from build123d import *

# Parameters (mm, degrees)
ESBO_O1_W                                = 150
ESBO_O1_H                                = 40
RESSALTO_EXTRUS_O1_DEPTH                 = 4
FILETE2_R                                = 15
BROCA_DE_ROSQUEAR_PARA_TARRAXA_DE_M201_D = 17.5


with BuildPart() as part:
    # Esboço1 → Ressalto-extrusão1 (new, symmetric)
    with BuildSketch(Plane.XY):
        with Locations((75, 20)):
            Rectangle(ESBO_O1_W, ESBO_O1_H)
    extrude(amount=RESSALTO_EXTRUS_O1_DEPTH, both=True)

    # Filete2
    filete2_edges = [part.edges().sort_by_distance(p)[0] for p in [
        (0, 0, 0),
        (0, 40, 0),
        (150, 40, 0),
        (150, 0, 0),
    ]]
    fillet(filete2_edges, radius=FILETE2_R)

    # Broca de rosquear para tarraxa de M201 (through all)
    with Locations(Plane.XY.offset(4)):
        with Locations((25, 20), (125, 20)):
            Hole(BROCA_DE_ROSQUEAR_PARA_TARRAXA_DE_M201_D / 2)


solid = part.part
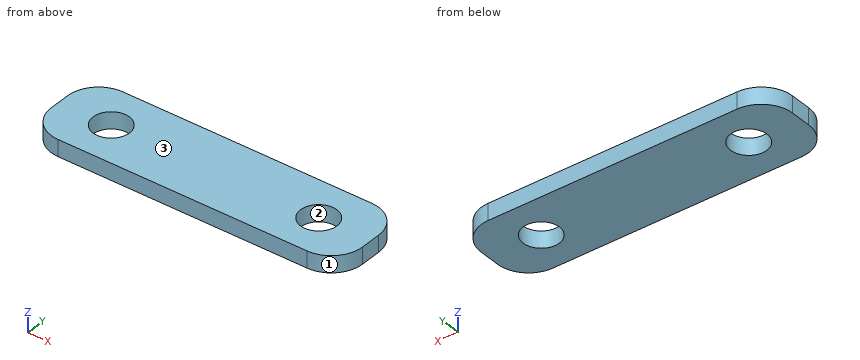
Could you check a few things on this model? Use its own coordinates, in mm. Face numbers are marked on the shaded views. Coordinates: 2 decimals unless noted, no trailing zeros. Order: outer loops, then holes, each group sorted by start corner. A loop starts at its lowest first (then second) coordinate and runs counter-clockwise, first axis right, second up. Notation, with made-up numbers: (-7, 23) - (47, 23) arc R22 ccw to (47, 56) - close; hole circle Ø11 at (50, -10). An arc over 180 degrees is marked (long way). Answer in a Markdown table with one row per item. Add a question column.
(1) I need wall thicknesses on L1, parallel to Y at x = 25, z = 1.5; L2, parallel to X at y = 25.5, z = -2.25; L3, parallel to X at y = 28, z = 0. Which ranges of each line are inside material? Lowest first, please.
(2) If we mould it in two halves opening along Y, with no side actions, what happens to the marked faces 1, 2 and 3? For each: released by +Y, released by -Y, zero draft, split by the parting line, or undercut.
(3) If we section it at A-A, the plane x = 125: Please give me the cut outline in (y, z), then the cut area to 3 significant figures.
(4) Will this pin go through, and if not, where does the flat tip stop? pin 1 (1 mm diameter, centred on y = 29.5, z = 1, fed in from -X).
(5) If we section it at B-B, the plane z = -0.5: Please give me the cut outline in (x, y), then the cut area to 3 significant figures.
(6) If we section it at C-C, the plane y = 20: Please give me the cut outline in (x, z).
(7) If we section it at D-D, the plane y = 3.5: Please give me the cut outline in (x, z).
Results are:
| question | item | result |
|---|---|---|
| 1 | L1 | y = 0 to 11.25, 28.75 to 40 |
| 1 | L2 | x = 0.01 to 18.19, 31.81 to 118.19, 131.81 to 149.99 |
| 1 | L3 | x = 0.3 to 21.46, 28.54 to 121.46, 128.54 to 149.7 |
| 2 | face 1 | released by -Y |
| 2 | face 2 | undercut |
| 2 | face 3 | zero draft |
| 3 | outline | (0, -4) - (11.25, -4) - (11.25, 4) - (0, 4) - close; (28.75, -4) - (40, -4) - (40, 4) - (28.75, 4) - close |
| 3 | area | 180 mm2 |
| 4 | pin 1 | stops at x = 0.54 |
| 5 | outline | (0, 15) arc R15 ccw to (15, 0) - (135, 0) arc R15 ccw to (150, 15) - (150, 25) arc R15 ccw to (135, 40) - (15, 40) arc R15 ccw to (0, 25) - close; hole circle Ø17.5 at (25, 20); hole circle Ø17.5 at (125, 20) |
| 5 | area | 5,330 mm2 |
| 6 | outline | (0, -4) - (16.25, -4) - (16.25, 4) - (0, 4) - close; (33.75, -4) - (116.25, -4) - (116.25, 4) - (33.75, 4) - close; (133.75, -4) - (150, -4) - (150, 4) - (133.75, 4) - close |
| 7 | outline | (5.37, -4) - (144.63, -4) - (144.63, 4) - (5.37, 4) - close |
